Input: part model. Units: mm. Frame: model coordinates. Face numbers are marked on the shaded views. A direction names the side the tool comes from. Give positions to 0.01 mm unless a question says otherwise; leave off trailing zeros. Order: outer loops, then holes, each group sorted by start corner. A loop starts at its lowest first (then second) coordinate and runs counter-clockwise, first axis right, second up. Notation, with made-up numbers: (63, 11) - (84, 11) arc R23 cw to (84, 41) - close; hole circle Ø3 at (-38.75, 40). An arc over 180 degrees is marked (long way). Use a Markdown table: item, result.
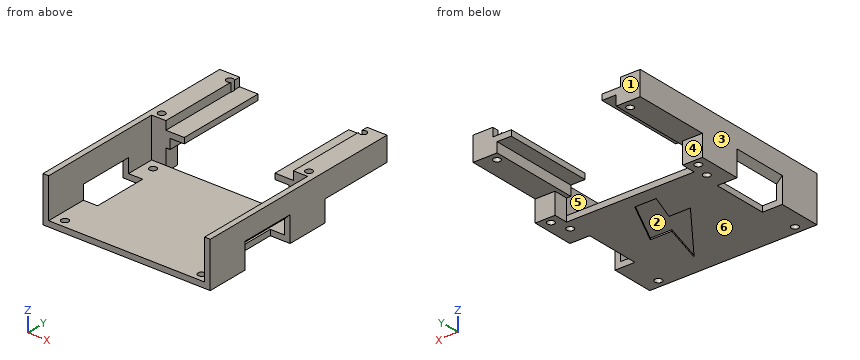
from build123d import *

# Parameters (mm, degrees)
BOSS_EXTRUDE1_DEPTH     = 44.5
SKETCH4_W               = 7
SKETCH4_H               = 9
BOSS_EXTRUDE3_DEPTH     = 5
SKETCH5_R               = 1.25
CUT_EXTRUDE3_DEPTH      = 78.538700015
BOSS_EXTRUDE4_DEPTH     = 3
SKETCH10_W              = 7
SKETCH10_H              = 19.5
CUT_EXTRUDE6_DEPTH      = 7
CHAMFER3_SIZE           = 2
CUT_EXTRUDE5_DEPTH      = 78.538700015
CUT_EXTRUDE5_DEPTH_BACK = 78.538700015
SKETCH9_W               = 59
SKETCH9_H               = 2
CUT_EXTRUDE7_DEPTH      = 0.5
SKETCH12_W              = 7
SKETCH12_H              = 2
SKETCH12_W_2            = 1.5
SKETCH12_H_2            = 3.5
SKETCH12_H_3            = 3
BOSS_EXTRUDE5_DEPTH     = 26.85
CUT_EXTRUDE4_START      = -16
CUT_EXTRUDE4_OUTLINE_R  = 1.25
CUT_EXTRUDE4_DEPTH      = 16
SKETCH12_4_W            = 1.5
SKETCH12_4_H            = 3.5
BOSS_EXTRUDE6_DEPTH     = 5


# Read off the part's stored shape, not the designer's step: Cut-Extrude4
with BuildPart() as part:
    # Sketch1 → Boss-Extrude1 (new body)
    with BuildSketch(Plane(origin=(0, 0, 0), x_dir=(1, 0, 0), z_dir=(0, 1, 0))):
        Polygon((0, 0), (2, 0), (2, 7), (57, 7), (57, 0), (59, 0), (59, 9), (0, 9), align=None)
    extrude(amount=BOSS_EXTRUDE1_DEPTH)

    # Sketch4 → Boss-Extrude3 (add)
    with BuildSketch(Plane(origin=(0, 44.5, 0), x_dir=(1, 0, 0), z_dir=(0, 1, 0))):
        with Locations((3.5, 4.5)):
            Rectangle(SKETCH4_W, SKETCH4_H)
        with Locations((55.5, 4.5)):
            Rectangle(SKETCH4_W, SKETCH4_H)
    extrude(amount=BOSS_EXTRUDE3_DEPTH)

    # Sketch5 → Cut-Extrude3 (cut, through all)
    with BuildSketch(Plane(origin=(0, 0, -9), x_dir=(-1, 0, 0), z_dir=(0, 0, -1))):
        with Locations((-55.5, 47)):
            Circle(SKETCH5_R)
        with Locations((-3.5, 47)):
            Circle(SKETCH5_R)
    extrude(amount=-CUT_EXTRUDE3_DEPTH, mode=Mode.SUBTRACT)

    # Sketch3 → Boss-Extrude4 (add)
    with BuildSketch(Plane(origin=(0, 0, -9), x_dir=(-1, 0, 0), z_dir=(0, 0, -1))):
        with BuildLine():
            ThreePointArc((1.75, 5), (1.184653197, 6.045825033), (0, 6.145643924))
            Line((0, 6.145643924), (0, 3.854356076))
            ThreePointArc((0, 3.854356076), (1.184653197, 3.954174967), (1.75, 5))
        make_face()
        with BuildLine():
            Line((-59, 3.854356076), (-59, 6.145643924))
            ThreePointArc((-59, 6.145643924), (-60.75, 5), (-59, 3.854356076))
        make_face()
    extrude(amount=BOSS_EXTRUDE4_DEPTH)


with BuildPart() as boss_extrude4_kept_piece:
    # of the separate pieces the step leaves, the one the design keeps (boss_extrude4_pieces_kept)
    add(part.part.solids().sort_by_distance((0, 49.5, 0))[0])

    # Mirror2: Boss-Extrude4 kept piece across plane


with BuildPart() as boss_extrude4_kept_piece_1:
    add(boss_extrude4_kept_piece.part)
    add(boss_extrude4_kept_piece.part.mirror(Plane.XY))

    # Sketch10 → Cut-Extrude6 (cut)
    with BuildSketch(Plane(origin=(0, 0, -9), x_dir=(-1, 0, 0), z_dir=(0, 0, -1))):
        with Locations((-55.5, 24.75)):
            Rectangle(SKETCH10_W, SKETCH10_H)
        with Locations((-3.5, 24.75)):
            Rectangle(SKETCH10_W, SKETCH10_H)
    extrude(amount=-CUT_EXTRUDE6_DEPTH, mode=Mode.SUBTRACT)

    # Chamfer3
    chamfer3_edges = [boss_extrude4_kept_piece_1.edges().sort_by_distance(p)[0] for p in [
        (0, 24.75, -2),
        (59, 24.75, -2),
    ]]
    chamfer(chamfer3_edges, length=CHAMFER3_SIZE - 0.0001)  # a hair under: the kernel refuses the full size

    # Sketch9 → Cut-Extrude5 (cut, two sides: drawn at the far end of the back side and taken through both)
    with BuildSketch(Plane.XZ.offset(-CUT_EXTRUDE5_DEPTH_BACK)):
        with Locations((29.5, 8)):
            Rectangle(SKETCH9_W, SKETCH9_H)
    extrude(amount=CUT_EXTRUDE5_DEPTH + CUT_EXTRUDE5_DEPTH_BACK, mode=Mode.SUBTRACT)

    # Sketch11 → Cut-Extrude7 (cut)
    with BuildSketch(Plane(origin=(0, 0, -9), x_dir=(-1, 0, 0), z_dir=(0, 0, -1))):
        Polygon((-32.1435681, 39.366852384), (-24.568842978, 39.366852384), (-28.293120049, 29.306670581), (-20.718394926, 29.306670581), (-37.51393239, 7.144924052), (-33.031231201, 22.264543319), (-40.605956323, 22.264543319), align=None)
    extrude(amount=-CUT_EXTRUDE7_DEPTH, mode=Mode.SUBTRACT)

    # Sketch12 → Boss-Extrude5 (add)
    with BuildSketch(Plane(origin=(0, 49.5, 0), x_dir=(1, 0, 0), z_dir=(0, 1, 0))):
        with Locations((55.5, -3)):
            Rectangle(SKETCH12_W, SKETCH12_H)
        Polygon((7, -2), (7, -4), (13.5, -4), (13.5, -2), (8.5, -2), align=None)
        Polygon((45.5, -2), (45.5, -4), (52, -4), (52, -2), (50.5, -2), align=None)
        with Locations((7.75, -0.25)):
            Rectangle(SKETCH12_W_2, SKETCH12_H_2)
        with Locations((3.5, -0.25)):
            Rectangle(SKETCH12_W, SKETCH12_H_2)
        with Locations((51.25, -0.25)):
            Rectangle(SKETCH12_W_2, SKETCH12_H_2)
        with Locations((55.5, -0.25)):
            Rectangle(SKETCH12_W, SKETCH12_H_2)
        with Locations((3.5, -3)):
            Rectangle(SKETCH12_W, SKETCH12_H)
        with Locations((3.5, -5.5)):
            Rectangle(SKETCH12_W, SKETCH12_H_3)
        with Locations((55.5, -5.5)):
            Rectangle(SKETCH12_W, SKETCH12_H_3)
    extrude(amount=BOSS_EXTRUDE5_DEPTH)

    # Cut-Extrude4 outline → Cut-Extrude4 (cut)
    with BuildSketch(Plane(origin=(0, 0, -9), x_dir=(-1, 0, 0), z_dir=(0, 0, -1)).offset(CUT_EXTRUDE4_START)):
        with Locations((-53, 73.35)):
            Circle(CUT_EXTRUDE4_OUTLINE_R)
        with Locations((-6, 73.35)):
            Circle(CUT_EXTRUDE4_OUTLINE_R)
        with Locations((-53.6, 40.95)):
            Circle(CUT_EXTRUDE4_OUTLINE_R)
        with Locations((-5.4, 40.95)):
            Circle(CUT_EXTRUDE4_OUTLINE_R)
        with Locations((-5.4, 2.9)):
            Circle(CUT_EXTRUDE4_OUTLINE_R)
        with Locations((-53.6, 2.9)):
            Circle(CUT_EXTRUDE4_OUTLINE_R)
    extrude(amount=CUT_EXTRUDE4_DEPTH, mode=Mode.SUBTRACT)

    # Sketch12<4> → Boss-Extrude6 (add)
    with BuildSketch(Plane(origin=(0, 49.5, 0), x_dir=(1, 0, 0), z_dir=(0, 1, 0))):
        Polygon((7, -2), (7, -4), (13.5, -4), (13.5, -2), (8.5, -2), align=None)
        Polygon((45.5, -2), (45.5, -4), (52, -4), (52, -2), (50.5, -2), align=None)
        with Locations((7.75, -0.25)):
            Rectangle(SKETCH12_4_W, SKETCH12_4_H)
        with Locations((51.25, -0.25)):
            Rectangle(SKETCH12_4_W, SKETCH12_4_H)
    extrude(amount=-BOSS_EXTRUDE6_DEPTH)


solid = boss_extrude4_kept_piece_1.part
1. Pin query (flat end, axial travel): pin 1 (1 mm diameter, centred on y = 28, z = -8, fed in from -X); pin 2 (6 mm diameter, centred on x = 43.5, z = -4.5, fed in from +Y); pin 3 (2 mm diameter, centred on x = 55.5, z = -6, fed in from +Y). Return the tip coordinate at first contact, or that it passes through.
Response:
| item | result |
|---|---|
| pin 1 | stops at x = 7 |
| pin 2 | stops at y = 44.5 |
| pin 3 | stops at y = 49.5 |
2. Set-up query: the marked faces 4, 5 and 6. Return all of +Z, -Z, +X, -X, +Y, -Y with unobstructed straight access to the full face (end or side cutting, diameter ignored); none if empty.
Response:
| item | result |
|---|---|
| face 4 | -Z, +X, -X, +Y |
| face 5 | +Z, -Y |
| face 6 | -Z, +X, -X, +Y, -Y |
3. Material intervals for line 1 along X through (y, z) = (47, -3.75); line 2 along X through (y, z) = (40.95, -8.6); line 3 along X through (y, z) = (47, -1.25), sorted ascending.
Response:
| item | result |
|---|---|
| line 1 | x = 0 to 2.25, 4.75 to 7, 52 to 54.25, 56.75 to 59 |
| line 2 | x = 0 to 4.15, 6.65 to 52.35, 54.85 to 59 |
| line 3 | x = 0 to 2.25, 4.75 to 8.5, 50.5 to 54.25, 56.75 to 59 |
4. Section query A-A (z = -3). Return loops of the section in (x, y).
Response:
| item | result |
|---|---|
| outline | (0, 0) - (2, 0) - (2, 15) - (0, 15) - close; (0, 34.5) - (2, 34.5) - (2, 44.5) - (7, 44.5) - (7, 49.5) - (0, 49.5) - close; (52, 44.5) - (57, 44.5) - (57, 34.5) - (59, 34.5) - (59, 49.5) - (52, 49.5) - close; (57, 0) - (59, 0) - (59, 15) - (57, 15) - close; hole circle Ø2.5 at (3.5, 47); hole circle Ø2.5 at (55.5, 47) |
5. Mould query, pull axis X, two halves, no side actions, for the marked faces 1, 2 and 3. Classes: pulls with the +X half, pulls with the -X half, needs draft (parallel to the pull), parting line crosses it, or undercut.
Response:
| item | result |
|---|---|
| face 1 | needs draft |
| face 2 | undercut |
| face 3 | pulls with the -X half |
6. Section query B-B (x = 12). Return loops of the section in (y, z), then the cut area to 3 significant figures.
Response:
| item | result |
|---|---|
| outline | (0, -9) - (44.5, -9) - (44.5, -7) - (0, -7) - close; (44.5, 2) - (76.35, 2) - (76.35, 4) - (44.5, 4) - close |
| area | 153 mm^2 |
7. Section query C-C (y = 2.9). Return loops of the section in (x, z).
Response:
| item | result |
|---|---|
| outline | (0, -9) - (4.15, -9) - (4.15, -7) - (2, -7) - (2, 7) - (0, 7) - close; (6.65, -9) - (52.35, -9) - (52.35, -7) - (6.65, -7) - close; (54.85, -9) - (59, -9) - (59, 7) - (57, 7) - (57, -7) - (54.85, -7) - close |
8. Section query D-D (y = 24.5). State how many separate pieces and enclosed holes the cut face has, then the cut area to 3 significant figures.
Response:
| item | result |
|---|---|
| separate pieces | 3 |
| enclosed holes | 0 |
| area | 114 mm^2 |
